Input: part model. Units: mm. Frame: model coordinates. A direction names the side the tool comes from. Coordinates: 2 decimals unless noted, no trailing zeros. Loops run counter-clockwise (first coordinate to the right, second up) from the corner with the lowest first, then second, coordinate; pieces in that order, holes last. Notation, with made-up numbers: (-33.75, 11.5) -> (-9.75, 11.5) arc R15 cw to (-9.75, 35.5) -> close; hole circle Ø1 at (-30, 71). An arc over 180 degrees is marked (long way). Answer as a JSON object with one key per item and string values.
from build123d import *

# Parameters (mm, degrees)
BOSS_EXTRUDE1_DEPTH = 33
SKETCH2_W           = 32
SKETCH2_H           = 33
BOSS_EXTRUDE2_DEPTH = 3
SKETCH3_R           = 1.9
CUT_EXTRUDE1_DEPTH  = 7
FILLET1_R           = 5
SKETCH5_R           = 2
BOSS_EXTRUDE3_DEPTH = 5
SKETCH6_W           = 32
SKETCH6_H           = 33
SKETCH6_W_2         = 28
SKETCH6_H_2         = 29
BOSS_EXTRUDE4_DEPTH = 5
BOSS_EXTRUDE5_DEPTH = 5
SKETCH7_R           = 0.75
SKETCH7_W           = 5
SKETCH7_H           = 119.688008906
CUT_EXTRUDE3_DEPTH  = 5
CUT_EXTRUDE4_DEPTH  = 53.302482054
CUT_EXTRUDE5_DEPTH  = 51.632111281
FILLET4_R           = 5


with BuildPart() as part:
    # Sketch1 → Boss-Extrude1 (new body)
    with BuildSketch(Plane(origin=(0, 0, 0), x_dir=(1, 0, 0), z_dir=(0, 1, 0))):
        Polygon((0, 0), (20, 0), (30.159835274, 17.597350892), (24.022012397, 21.141024582), align=None)
    extrude(amount=BOSS_EXTRUDE1_DEPTH)

    # Sketch2 → Boss-Extrude2 (add)
    with BuildSketch(Plane(origin=(0, 0, 0), x_dir=(0.7506878874077226, 0, -0.660657018201828), z_dir=(0.660657018201828, 0, 0.7506878874077226))):
        with Locations((16, 16.5)):
            Rectangle(SKETCH2_W, SKETCH2_H)
    extrude(amount=-BOSS_EXTRUDE2_DEPTH)

    # Sketch3 → Cut-Extrude1 (cut)
    with BuildSketch(Plane(origin=(30, 0, 0), x_dir=(-1, 0, 0), z_dir=(0, 0, -1))):
        with Locations((18, 29)):
            Circle(SKETCH3_R)
        with Locations((18, 4)):
            Circle(SKETCH3_R)
    extrude(amount=CUT_EXTRUDE1_DEPTH, mode=Mode.SUBTRACT)

    # Fillet1
    fillet1_edges = [part.edges().sort_by_distance(p)[0] for p in [
        (20, 16.5, 0),
    ]]
    fillet(fillet1_edges, radius=FILLET1_R)

    # Sketch5 → Boss-Extrude3 (add)
    with BuildSketch(Plane(origin=(-1.981971055, 0, -2.252063662), x_dir=(-0.7506878874077226, 0, 0.660657018201828), z_dir=(-0.660657018201828, 0, -0.7506878874077226))):
        with Locations((-28.3, 28.4)):
            Circle(SKETCH5_R)
        with Locations((-3.7, 28.4)):
            Circle(SKETCH5_R)
        with Locations((-28.3, 4.6)):
            Circle(SKETCH5_R)
        with Locations((-3.7, 4.6)):
            Circle(SKETCH5_R)
    extrude(amount=BOSS_EXTRUDE3_DEPTH)

    # Sketch6 → Boss-Extrude4 (add)
    with BuildSketch(Plane(origin=(-1.981971055, 0, -2.252063662), x_dir=(-0.7506878874077226, 0, 0.660657018201828), z_dir=(-0.660657018201828, 0, -0.7506878874077226))):
        with Locations((-16, 16.5)):
            Rectangle(SKETCH6_W, SKETCH6_H)
        with Locations((-16, 16.5)):
            Rectangle(SKETCH6_W_2, SKETCH6_H_2, mode=Mode.SUBTRACT)
    extrude(amount=BOSS_EXTRUDE4_DEPTH)

    # Sketch9 → Boss-Extrude5 (add)
    with BuildSketch(Plane(origin=(-1.981971055, 0, -2.252063662), x_dir=(-0.7506878874077226, 0, 0.660657018201828), z_dir=(-0.660657018201828, 0, -0.7506878874077226))):
        Polygon((-28.3, 26.4), (-30, 26.4), (-30, 31), (-26.3, 31), (-26.3, 28.4), align=None)
        Polygon((-5.7, 28.4), (-5.7, 31), (-2, 31), (-2, 26.4), (-3.7, 26.4), align=None)
        Polygon((-3.7, 6.6), (-2, 6.6), (-2, 2), (-5.7, 2), (-5.7, 4.6), align=None)
        Polygon((-28.3, 6.6), (-30, 6.6), (-30, 2), (-26.3, 2), (-26.3, 4.6), align=None)
    extrude(amount=BOSS_EXTRUDE5_DEPTH)

    # Sketch7 → Cut-Extrude3 (cut)
    with BuildSketch(Plane(origin=(-5.285256146, 0, -6.005503099), x_dir=(-0.7506878874077226, 0, 0.660657018201828), z_dir=(-0.660657018201828, 0, -0.7506878874077226))):
        with Locations((-28.3, 28.4)):
            Circle(SKETCH7_R)
        with Locations((-3.7, 28.4)):
            Circle(SKETCH7_R)
        with Locations((-3.7, 4.6)):
            Circle(SKETCH7_R)
        with Locations((-28.3, 4.6)):
            Circle(SKETCH7_R)
        with Locations((-16, 31)):
            Rectangle(SKETCH7_W, SKETCH7_H)
    extrude(amount=-CUT_EXTRUDE3_DEPTH, mode=Mode.SUBTRACT)

    # Sketch8 → Cut-Extrude4 (cut, through all)
    with BuildSketch(Plane(origin=(0, 33, 0), x_dir=(1, 0, 0), z_dir=(0, 1, 0))):
        Polygon((17.745348673, 28.950001735), (16.878144986, 39.625600728), (45.212516216, 18.101512889), (33.036600924, 2.073102927), align=None)
    extrude(amount=-CUT_EXTRUDE4_DEPTH, mode=Mode.SUBTRACT)

    # Sketch10 → Cut-Extrude5 (cut, through all)
    with BuildSketch(Plane(origin=(0, 33, 0), x_dir=(1, 0, 0), z_dir=(0, 1, 0))):
        Polygon((22.997492955, 19.718491584), (15.018022413, 13.241165816), (22.396735909, 4.151268367), (32.809004156, 12.603414793), align=None)
    extrude(amount=-CUT_EXTRUDE5_DEPTH, mode=Mode.SUBTRACT)

    # Fillet4
    # the kernel refuses this fillet: 5 mm, written as the material it adds along each edge
    with BuildSketch(Plane(origin=(15.018022413, 33, -13.241165816), x_dir=(0.7763993545799179, 0, -0.6302412571451403), z_dir=(0, -1, 0))) as fillet4_piece_1:
        with BuildLine():
            CenterArc((FILLET4_R, FILLET4_R), FILLET4_R, 180, 90)
            Line((0, FILLET4_R), (0, 0))
            Line((0, 0), (FILLET4_R, 0))
        make_face()
    extrude(amount=33)
    # the kernel refuses this fillet: 5 mm, written as the material it takes off along each edge
    with BuildSketch(Plane(origin=(22.396735909, 40.861690342, -4.151268367), x_dir=(-0.6302412571451408, 0, -0.7763993545799174), z_dir=(0, -1, 0))) as fillet4_2_piece_1:
        with BuildLine():
            CenterArc((3.144676137, -5), FILLET4_R, 90, 49.922525522)
            Line((-0.681196741, -1.780885723), (0, 0))
            Line((0, 0), (3.144676137, 0))
        make_face()
    extrude(amount=48.723380684, mode=Mode.SUBTRACT)
    with BuildSketch(Plane(origin=(22.997492955, 43.594997798, -19.718491584), x_dir=(-0.4945052818029634, 0, -0.8691746235762823), z_dir=(0, -1, 0))) as fillet4_2_piece_2:
        with BuildLine():
            CenterArc((FILLET4_R * 0.847599823854, -FILLET4_R), FILLET4_R, 90, 80.569209056)
            Line((-FILLET4_R * 0.138884423377, -FILLET4_R * 0.836143874187), (0, 0))
            Line((0, 0), (FILLET4_R * 0.847599823854, 0))
        make_face()
    extrude(amount=54.189995596, mode=Mode.SUBTRACT)
    with BuildSketch(Plane(origin=(0, -5.650533789, 0), x_dir=(1, 0, 0), z_dir=(0, 1, 0))) as fillet4_2_piece_3:
        with BuildLine():
            CenterArc((FILLET4_R * 0.452042703087, FILLET4_R), FILLET4_R, 221.35, 48.65)
            Line((-FILLET4_R * 0.298645184321, FILLET4_R * 0.339342981798), (0, 0))
            Line((0, 0), (FILLET4_R * 0.452042703087, 0))
        make_face()
    extrude(amount=44.301067577, mode=Mode.SUBTRACT)


solid = part.part
1. Line query: line 1 along Y through (x, z) = (12, -2.5); line 2 along Y through (x, z) = (4.25, -11.5); line 3 along Z through (x, y) = (20.25, 19). Output: solid intervals per line, ascending.
Reply:
{"line 1": "y = 0 to 2.1, 5.9 to 27.1, 30.9 to 33", "line 2": "y = 0 to 2, 31 to 33", "line 3": "z = -24.55 to -22.4, -21.82 to -17.56, -6.8 to -1.11"}
2. Mould query, pull axis Y, two halves, no side actions, for faces 4 (the face through (0.8, 4.6, -4.7)), 5 (the face through (17.4, 17.8, -25.97)). Classes: pulls with the +Y half, pulls with the -Y half, needs draft (parallel to the pull), parting line crosses it, or undercut.
Reply:
{"face 4": "undercut", "face 5": "needs draft"}
3. Section query A-A (y = 15). Return loops of the section in (x, z).
Reply:
{"outline": "(-5.29, -6.01) -> (-3.78, -7.33) -> (-0.48, -3.57) -> (20.54, -22.07) -> (17.24, -25.83) -> (18.74, -27.15) -> (18.83, -27.04) -> (20.9, -23.4) arc R5 ccw to (19.71, -17.05) -> (18.9, -16.39) arc R5 cw to (18.17, -9.36) -> (20.41, -6.59) arc R5 ccw to (21.44, -2.5) arc R5 ccw to (17.11, 0) -> (2.26, 0) arc R5 ccw to (-1.49, -1.7) -> close"}
4. Section query C-C (y = 3). Return loops of the section in (x, z).
Reply:
{"outline": "(-5.29, -6.01) -> (-1.01, -9.77) -> (2.3, -6.02) -> (17.76, -19.63) -> (14.46, -23.38) -> (18.74, -27.15) -> (18.83, -27.04) -> (20.9, -23.4) arc R5 ccw to (19.71, -17.05) -> (18.9, -16.39) arc R5 cw to (18.17, -9.36) -> (20.41, -6.59) arc R5 ccw to (21.44, -2.5) arc R5 ccw to (17.11, 0) -> (13.62, 0) -> (13.62, -7) -> (10.38, -7) -> (10.38, 0) -> (2.26, 0) arc R5 ccw to (-1.49, -1.7) -> close"}
5. Access query for faces 1 (the face through (13, 2, -19)), 2 (the face through (6.48, 0.99, -13.07)), 3 (the face through (0.8, 28.4, -4.7)). Directions: +Z, -Z, +X, -X, +Y, -Y. A direction counts if a zero-diameter tool reaches every point of the face in a straight line with its end or side. Return the directions, or none.
Reply:
{"face 1": "-X", "face 2": "-Z, +Y, -Y", "face 3": "none"}
6. Section query B-B (x = 5.5). Return loops of the section in (y, z), plus the area to 3 significant figures.
Reply:
{"outline": "(0, -14.18) -> (2, -14.18) -> (2, -8.84) -> (31, -8.84) -> (31, -14.18) -> (33, -14.18) -> (33, 0) -> (0, 0) -> close", "area": "313 mm2"}
7. Pin query (flat end, axial travel): P1, Ø2, axis at y = 15, z = -20.5, coming from the -X side; P2, Ø1, axis at y = 19.5, z = -17, coming from the -X side; P3, Ø4, axis at x = 11.5, y = 29, coming from the +Z side; P4, Ø2, axis at x = 6.5, y = 9.5, coming from the -Z side. Return the tip coordinate at first contact, or that it passes through.
Reply:
{"P1": "stops at x = 17.62", "P2": "stops at x = 14.21", "P3": "stops at z = 0", "P4": "stops at z = -10.6"}
